Autodesk Inventor part; units mm, degrees
ref_plane "YZ Plane" through (0, 0, 0) normal (1, 0, 0) x (0, 1, 0)
ref_plane "XZ Plane" through (0, 0, 0) normal (0, 1, 0) x (-1, 0, 0)
ref_plane "XY Plane" through (0, 0, 0) normal (0, 0, 1) x (1, 0, 0)
sketch "Sketch1" plane through (0, 0, 0) normal (0, 0, 1) x (1, 0, 0)
  line L0 (0, 0) -> (35, 0)
  line L1 (55, 20) -> (55, 120) construction
  line L2 (52.2444, 206.3696) -> (25, 285)
  line L3 (25, 285) -> (25, 305)
  line L4 (25, 305) -> (0, 305)
  line L5 (0, 305) -> (0, 0)
  arc A0 (55, 190) -> (52.2444, 206.3696) centre (5, 190) ccw
  arc A1 (35, 0) -> (55, 20) centre (35, 20) ccw
  line L6 (55, 120) -> (50, 106.3786)
  line L7 (50, 106.3786) -> (50, 33.6214)
  line L8 (50, 33.6214) -> (55, 20)
  line L9 (55, 120) -> (55, 190)
  point P0 (55, 0)
  dimension "d1" = 55
  dimension "d4" = 50
  dimension "d6" = 25
  dimension "d7" = 20
  dimension "d8" = 115
  dimension "d9" = 20
  dimension "d10" = 70
  dimension "d11" = 120
  dimension "d12" = 5
revolve "Revolution1" add sketch "Sketch1" angle 360 about axis through (0, 305, 0) along (0, -1, 0)
properties part number "2L bottle"
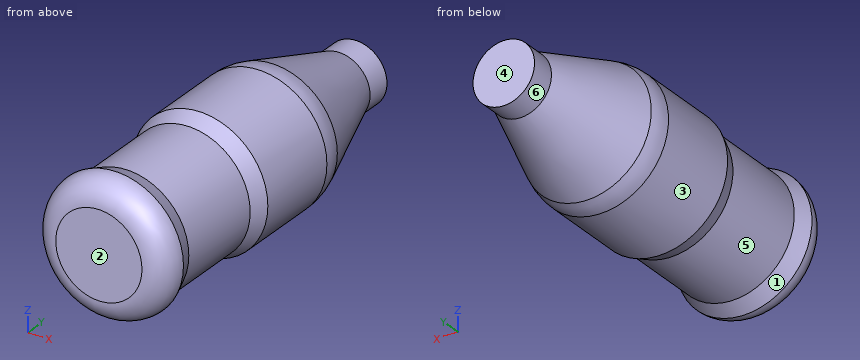
Verification items for the finished model (mm, model axes). Face numbers are marked on the shaded views. A direction names the side the tool comes from. Coordinates: 2 decimals unless noted, no trailing zeros. Order: outer loops, then holes, each group sorted by start corner. A loop starts at its lowest first (then second) coordinate and runs counter-clockwise, first axis right, second up.
1. Set-up check for the marked faces 5 and 6: record each of +Z, -Z, +X, -X, +Y, -Y from which the full face is reachable in a straight line by a thin tool's end or side.
Results found:
face 5: none
face 6: +Y
2. Sectioned sample at B-B, the plane y = 171. Record the cut outline in (x, z).
Results found:
outline: circle Ø110 at (0, 0)
3. Release check for a two-part mould opening along Y. For the marked faces 1, 2, 3 and 4 record: +Y half, -Y half, draft (parallel to the pull), parting line (faces both ways), or undercut.
Results found:
face 1: undercut
face 2: -Y half
face 3: draft
face 4: +Y half
4. Sectioned sample at A-A, the plane y = 216. Record the cut outline in (x, z).
Results found:
outline: circle Ø97.82 at (0, 0)
5. Go/stop test with flat-tipped pins: pin 1 Ø10 at (x, y) = (-23.5, 95.5) entering from +Z; pin 2 Ø3 at (y, z) = (121.5, 19) entering from +X; pin 3 Ø3 at (x, y) = (-27.5, 83) entering from -Z. Record where each tip stops, or that it passes through.
Results found:
pin 1: stops at z = 46.45
pin 2: stops at x = 52.14
pin 3: stops at z = -42.71
6. Scan lines: line 1 (Y direction, x = 33, z = -40); line 2 (Y direction, x = 28, z = 42); line 3 (X direction, y = 18, z = 47). Record each from-to range of solid material in increasing order.
Results found:
line 1: y = 9.23 to 28.57, 111.43 to 207.49
line 2: y = 7.33 to 32.32, 107.68 to 211.47
line 3: x = -28.37 to 28.37
